The model under review builds one solid part; all positions refer to its coordinate system, in mm. A direction names the side the tool comes from. Round coordinates to 2 decimals unless told otherwise and drop trailing zeros. Loops run counter-clockwise (first coordinate to the right, second up) from the corner with the lowest first, then second, coordinate; pieces in that order, holes last. Notation, with made-up numbers: (-7, 15) -> (40, 15) arc R20 cw to (40, 44) -> close; hole circle Ø5 at (-27.75, -34.5). An arc over 180 degrees is marked (long way). Use a Markdown table: item, result. Add a question column.
1) Consider section A-A on x = 60. Give the boundary of the cut face in (y, z).
2) Mouldability with a two-part tool opening along Y and no side actions: class faces 1 (the cylindrical face through (-89.97, 1.32, 37.67)), 2 (the flat face through (-7, -50, 25)), 3 (the flat face through (-7, 1, 50)) as released by +Y, released by -Y, zero draft, split by the parting line, or undercut.
3) Wall thickness on probe 1 along Y at (x, z) = (-180, 42); probe 2 along Z at (x, y) = (-48, -4); probe 3 along Y at (x, z) = (-186.5, 43.5): over which ranges is each line inside the solid? List them lowest first.
4) Consider section B-B on x = 170. Give the boundary of the cut face in (y, z), plus the area to 3 significant figures.
5) For faces 4 (the cylindrical face through (208.615, 9.011, 37.675)), 5 (the flat face through (-7, 1, 0)), list the 3-axis set-ups (+Z, -Z, +X, -X, +Y, -Y) from which the entire face can be reached by the end or side of a thin tool; tool diameter is ignored.
from build123d import *

# Parameters (mm, degrees)
SKETCH1_W           = 900
SKETCH1_H           = 100
BOSS_EXTRUDE1_DEPTH = 50
SKETCH2_R           = 30
SKETCH2_W           = 40
SKETCH2_H           = 20
CUT_EXTRUDE1_DEPTH  = 25
SKETCH3_W           = 50
SKETCH3_H           = 50
BOSS_EXTRUDE3_DEPTH = 100


with BuildPart() as part:
    # Sketch1 → Boss-Extrude1 (new body)
    with BuildSketch(Plane.XY):
        Rectangle(SKETCH1_W, SKETCH1_H)
    extrude(amount=BOSS_EXTRUDE1_DEPTH)

    # Sketch2 → Cut-Extrude1 (cut)
    with BuildSketch(Plane.XY.offset(50)):
        with Locations((-300, 0)):
            Circle(SKETCH2_R)
        with Locations((-180, 0)):
            Circle(SKETCH2_R)
        with Locations((-60, 0)):
            Circle(SKETCH2_R)
        with Locations((60, 0)):
            Circle(SKETCH2_R)
        with Locations((180, 0)):
            Circle(SKETCH2_R)
        with Locations((300, 0)):
            Circle(SKETCH2_R)
        with Locations((400, 0)):
            Rectangle(SKETCH2_W, SKETCH2_H)
        with Locations((-400, 0)):
            Rectangle(SKETCH2_W, SKETCH2_H)
    extrude(amount=-CUT_EXTRUDE1_DEPTH, mode=Mode.SUBTRACT)

    # Sketch3 → Boss-Extrude3 (add)
    with BuildSketch(Plane(origin=(0, 50, 0), x_dir=(1, 0, 0), z_dir=(0, 1, 0))):
        with Locations((475, -25)):
            Rectangle(SKETCH3_W, SKETCH3_H)
        with Locations((-475, -25)):
            Rectangle(SKETCH3_W, SKETCH3_H)
    extrude(amount=-BOSS_EXTRUDE3_DEPTH)


solid = part.part
Result set:
| question | item | result |
|---|---|---|
| 1 | outline | (-50, 0) -> (50, 0) -> (50, 50) -> (30, 50) -> (30, 25) -> (-30, 25) -> (-30, 50) -> (-50, 50) -> close |
| 2 | face 1 | undercut |
| 2 | face 2 | released by -Y |
| 2 | face 3 | zero draft |
| 3 | probe 1 | -50 to -30, 30 to 50 |
| 3 | probe 2 | 0 to 25 |
| 3 | probe 3 | -50 to -29.29, 29.29 to 50 |
| 4 | outline | (-50, 0) -> (50, 0) -> (50, 50) -> (28.28, 50) -> (28.28, 25) -> (-28.28, 25) -> (-28.28, 50) -> (-50, 50) -> close |
| 4 | area | 3,590 mm2 |
| 5 | face 4 | +Z |
| 5 | face 5 | -Z, +X, -X, +Y, -Y |
